from build123d import *

# Parameters (mm, degrees)
BASE_FLANGE1_START = -279.99988
BASE_FLANGE1_DEPTH = 559.99976
SKETCH8_W          = 292.444779068
SKETCH8_H          = 100
CUT_EXTRUDE1_DEPTH = 898.788870169


# Sheet-metal steps are written as plain solids
with BuildPart() as part:
    # Sketch3 → Base-Flange1 (new body)
    with BuildSketch(Plane(origin=(-250, -934.739885498, -1517.780517475), x_dir=(0, 0, -1), z_dir=(1, 0, 0)).offset(BASE_FLANGE1_START)):
        with BuildLine():
            Line((-1517.780517475, 789.739945498), (-1517.780517475, 919.739945498))
            Line((-1517.780517475, 919.739945498), (-1517.780517475, 946.019792244))
            ThreePointArc((-1517.780517475, 946.019792244), (-1516.791982116, 949.004444892), (-1514.217256902, 950.80892367))
            Line((-1514.217256902, 950.80892367), (-1468.483412721, 964.529076924))
            ThreePointArc((-1468.483412721, 964.529076924), (-1467.772739017, 964.686947476), (-1467.046673293, 964.739945498))
            Line((-1467.046673293, 964.739945498), (-868.514361656, 964.739945498))
            ThreePointArc((-868.514361656, 964.739945498), (-867.788295933, 964.686947476), (-867.077622228, 964.529076924))
            Line((-867.077622228, 964.529076924), (-821.343778047, 950.80892367))
            ThreePointArc((-821.343778047, 950.80892367), (-818.769052833, 949.004444892), (-817.780517475, 946.019792244))
            Line((-817.780517475, 946.019792244), (-817.780517475, 919.739945498))
            Line((-817.780517475, 919.739945498), (-812.780517475, 919.739945498))
            Line((-812.780517475, 919.739945498), (-812.780517475, 946.019792244))
            ThreePointArc((-812.780517475, 946.019792244), (-814.757588192, 951.98909754), (-819.907038619, 955.598055096))
            Line((-819.907038619, 955.598055096), (-865.6408828, 969.318208351))
            ThreePointArc((-865.6408828, 969.31820835), (-867.062230209, 969.633949453), (-868.514361657, 969.739945498))
            Line((-868.514361656, 969.739945498), (-1467.046673293, 969.739945498))
            ThreePointArc((-1467.046673294, 969.739945498), (-1468.49880474, 969.633949453), (-1469.920152148, 969.318208351))
            Line((-1469.920152149, 969.318208351), (-1515.65399633, 955.598055096))
            ThreePointArc((-1515.65399633, 955.598055096), (-1520.803446757, 951.98909754), (-1522.780517475, 946.019792244))
            Line((-1522.780517475, 946.019792244), (-1522.780517475, 919.739945498))
            Line((-1522.780517475, 919.739945498), (-1522.780517475, 789.739945498))
            Line((-1522.780517475, 789.739945498), (-1517.780517475, 789.739945498))
        make_face()
    extrude(amount=BASE_FLANGE1_DEPTH)

    # Sketch8 → Cut-Extrude1 (cut, through all)
    with BuildSketch(Plane.XY.offset(5)):
        with Locations((-250, -94.99994)):
            Rectangle(SKETCH8_W, SKETCH8_H)
    extrude(amount=-CUT_EXTRUDE1_DEPTH, mode=Mode.SUBTRACT)


solid = part.part
For this review, take the finished solid that the model builds, in its own axes (mm). A direction names the side the tool comes from. Give positions to 0.01 mm unless a question says otherwise; leave off trailing zeros. Order: outer loops, then holes, each group sorted by start corner. A loop starts at its lowest first (then second) coordinate and runs counter-clockwise, first axis right, second up. Notation, with made-up numbers: (-39, 10.25) - (6, 10.25) arc R30 ccw to (6, 38.25) - close; hole circle Ø10 at (59.5, 52). An arc over 180 degrees is marked (long way). Answer as a JSON object with one key per item and string values. Group by question number.
Item 1: Take a section at C-C on z = -422. Give the boundary of the cut face in (x, y), and give its area (3 significant figures).
Item 2: Clearance check with flat-ended pins moving along their axes: pin 1 Ø4 at (x, z) = (-219.5, 1.5) entering from -Y; pin 2 Ø1.5 at (x, z) = (-206, -702.5) entering from -Y; pin 3 Ø3 at (x, z) = (-42, -571) entering from -Y. State where each tip first meets the part, or that it passes through.
Item 3: Machinability: for faces 4 (the flat face through (-254, 35, -354)), 5 (the flat face through (-253.92, 22.833, -26.11)), which of the approach directions +Z, -Z, +X, -X, +Y, -Y give a long, thin tool a straight path to every point of the face, cutting with its end or side? Answer none if there is none.
Item 4: Wall thickness on line 1 along Z through (x, y) = (-354.5, -3.5); line 2 along Z through (x, y) = (-404, -124.5); line 3 along Y through (x, z) = (-54, -313): over which ranges is each line inside the solid? List them lowest first.
Item 5: Draft analysis for pull direction Z (two halves, no side actions). For faces 1 (the flat face through (-253.92, 23.025, -673.25)), 2 (the flat face through (-530, 32, -348)), 3 (the flat face through (-253.92, 27.814, -25.314)), state which applies: pulls with the +Z half, pulls with the -Z half, needs draft (parallel to the pull), parting line crosses it, or undercut.
Item 6: Take a section at D-D on x = -39. Give the boundary of the cut face in (y, z), and give its area (3 significant figures).
Item 7: Take a section at A-A on y = -93. Give the boundary of the cut face in (x, z).
Item 8: Take a section at B-B on x = -341. Give the boundary of the cut face in (y, z).
Reported:
{
 "1": {"outline": "(-530, 30) - (30, 30) - (30, 35) - (-530, 35) - close", "area": "2,800 mm^2"},
 "2": {"pin 1": "y = -45", "pin 2": "y = -15", "pin 3": "y = 30"},
 "3": {"face 4": "+Z, -Z, +X, -X, +Y", "face 5": "+X, -X, -Y"},
 "4": {"line 1": "-705 to -700, 0 to 5", "line 2": "0 to 5", "line 3": "30 to 35"},
 "5": {"face 1": "undercut", "face 2": "needs draft", "face 3": "pulls with the +Z half"},
 "6": {"outline": "(-145, 0) - (11.28, 0) arc R5 cw to (16.07, -3.56) - (29.79, -49.3) arc R5 cw to (30, -50.73) - (30, -649.27) arc R5 cw to (29.79, -650.7) - (16.07, -696.44) arc R5 cw to (11.28, -700) - (-15, -700) - (-15, -705) - (11.28, -705) arc R10 ccw to (20.86, -697.87) - (34.58, -652.14) arc R10 ccw to (35, -649.27) - (35, -50.73) arc R10 ccw to (34.58, -47.86) - (20.86, -2.13) arc R10 ccw to (11.28, 5) - (-145, 5) - close", "area": "4,500 mm^2"},
 "7": {"outline": "(-530, 0) - (-396.22, 0) - (-396.22, 5) - (-530, 5) - close; (-103.78, 0) - (30, 0) - (30, 5) - (-103.78, 5) - close"},
 "8": {"outline": "(-45, 0) - (11.28, 0) arc R5 cw to (16.07, -3.56) - (29.79, -49.3) arc R5 cw to (30, -50.73) - (30, -649.27) arc R5 cw to (29.79, -650.7) - (16.07, -696.44) arc R5 cw to (11.28, -700) - (-15, -700) - (-15, -705) - (11.28, -705) arc R10 ccw to (20.86, -697.87) - (34.58, -652.14) arc R10 ccw to (35, -649.27) - (35, -50.73) arc R10 ccw to (34.58, -47.86) - (20.86, -2.13) arc R10 ccw to (11.28, 5) - (-45, 5) - close"}
}
